from build123d import *

# Parameters (mm, degrees)
F1_DEPTH = 81.026
F2_W     = 28.9863510989
F2_H     = 31.3605703413
F3_DEPTH = 60.198


with BuildPart() as f1:
    # F0 (on Front) → F1 (new body)
    with BuildSketch(Plane.XZ):
        Polygon((-12.2977383435, 51.6691952944), (1.6879233299, 0), (59.5596246421, 27.5620631874), align=None)
    extrude(amount=F1_DEPTH)

    # F2 (on face) → F3 (join)
    with BuildSketch(Plane(origin=(14.3365736593, 0, 42.733759156), x_dir=(0.9480692853, 0, -0.3180638776), z_dir=(0.3180638776, 0, 0.9480692853))):
        with Locations((9.7663637716, -36.5160163492)):
            Rectangle(F2_W, F2_H)
    extrude(amount=F3_DEPTH)


solid = f1.part
Source: CAD feature listing. Evaluate the final solid. Frame: model axes, mm. A direction names the side the tool comes from. Round coordinates to 2 decimals unless told otherwise and drop trailing zeros. Loops run counter-clockwise (first coordinate to the right, second up) from the corner with the lowest first, then second, coordinate; pieces in that order, holes last.
Q1. Section B-B, the plane z = 46. Return loops of the section in (x, y).
Q2. Section A-A, the plane y = -50.5. Return loops of the section in (x, z).
Q3. Ray query, line 1 (Y direction, x = 36.5, z = 44); line 2 (X direction, y = -40.5, z = 62); line 3 (Z direction, x = 54, y = -68). Return the intervals inside material, ascending.
Q4. Section D-D, the plane x = 31. Return loops of the section in (y, z), plus the area to 3 significant figures.
Q5. Access query for faces 5 (the face through (33, -20.836, 68)), 6 (the face through (33, -52.196, 68)), 7 (the face through (15, -81.026, 26)). Directions: +Z, -Z, +X, -X, +Y, -Y. A direction counts if a zero-diameter tool reaches every point of the face in a straight line with its end or side. Return the directions, or none.
Q6. Mould query, pull axis X, two halves, no side actions, for faces 1 (the face through (15, 0, 26)), 2 (the face through (40.1, -39.95, 34.09)), 3 (the face through (-5.403, -39.946, 26.196)), 4 (the face through (46.776, -36.736, 63.154)). Classes: pulls with the +X half, pulls with the -X half, needs draft (parallel to the pull), parting line crosses it, or undercut.
Q7. First-contact query: P1, Ø10, axis at x = 44.5, y = -64.5, coming from the +Z side; P2, Ø2, axis at y = -33, z = 71.5, coming from the +X side; P3, Ø12, axis at x = 31, z = 70.5, coming from the +Y side. Flat tips, straight axial feed; report the tip coordinate or a pass-through.
Q8. Section C-C, the plane x = 50.5. Return loops of the section in (y, z).
Solutions:
1. outline: (-10.76, -81.03) - (4.6, -81.03) - (4.6, 0) - (-10.76, 0) - close; (10.45, -52.2) - (41.02, -52.2) - (41.02, -20.84) - (10.45, -20.84) - close
2. outline: (-12.3, 51.67) - (1.69, 0) - (59.56, 27.56) - (37.34, 35.02) - (56.48, 92.09) - (29, 101.31) - (9.86, 44.24) - close
3. line 1: y = -52.2 to -20.84
3. line 2: x = 15.81 to 46.39
3. line 3: z = 24.91 to 29.43
4. outline: (-81.03, 13.96) - (0, 13.96) - (0, 37.14) - (-20.84, 37.14) - (-20.84, 100.64) - (-52.2, 100.64) - (-52.2, 37.14) - (-81.03, 37.14) - close
4. area: 3,870 mm2
5. face 5: +Z, +X, +Y
5. face 6: +Z, +X, -Y
5. face 7: +Z, -Z, +X, -X, -Y
6. face 1: needs draft
6. face 2: undercut
6. face 3: pulls with the -X half
6. face 4: pulls with the +X half
7. P1: stops at z = 34.29
7. P2: stops at x = 49.91
7. P3: stops at y = -20.84
8. outline: (-81.03, 23.25) - (0, 23.25) - (0, 30.6) - (-81.03, 30.6) - close; (-52.2, 74.26) - (-20.84, 74.26) - (-20.84, 94.1) - (-52.2, 94.1) - close
